```python
from build123d import *

# Parameters (mm, degrees)
SKETCH1_R           = 2.475
EXTRUDE1_DEPTH      = 17.8
SKETCH2_OUTSIDE_W   = 10.776
SKETCH2_OUTSIDE_H   = 10.776
SKETCH2_OUTSIDE_W_2 = 2.9
SKETCH2_OUTSIDE_H_2 = 7
EXTRUDE2_DEPTH      = 6
CHAMFER1_SIZE       = 0.3
CHAMFER2_SIZE       = 0.3


with BuildPart() as part:
    # Sketch1 → Extrude1 (new body)
    with BuildSketch(Plane.XY):
        Circle(SKETCH1_R)
    extrude(amount=EXTRUDE1_DEPTH)

    # Sketch2 outside → Extrude2 (cut)
    with BuildSketch(Plane.XY.offset(17.8)):
        Rectangle(SKETCH2_OUTSIDE_W, SKETCH2_OUTSIDE_H)
        Rectangle(SKETCH2_OUTSIDE_W_2, SKETCH2_OUTSIDE_H_2, mode=Mode.SUBTRACT)
    extrude(amount=-EXTRUDE2_DEPTH, mode=Mode.SUBTRACT)

    # Chamfer1
    chamfer1_edges = [part.edges().sort_by_distance(p)[0] for p in [
        (0, 2.475, 17.8),
        (0, -2.475, 17.8),
    ]]
    chamfer(chamfer1_edges, length=CHAMFER1_SIZE)

    # Chamfer2
    chamfer2_edges = [part.edges().sort_by_distance(p)[0] for p in [
        (-1.45, 0, 11.8),
        (1.45, 0, 11.8),
    ]]
    chamfer(chamfer2_edges, length=CHAMFER2_SIZE)


solid = part.part
```
Input: part model. Units: mm. Frame: model coordinates. A direction names the side the tool comes from. Round coordinates to 2 decimals unless told otherwise and drop trailing zeros. Loops run counter-clockwise (first coordinate to the right, second up) from the corner with the lowest first, then second, coordinate; pieces in that order, holes last. Notation, with made-up numbers: (48, 74.5) -> (97, 74.5) arc R15 ccw to (97, 82.5) -> close; hole circle Ø10 at (15, -5). An arc over 180 degrees is marked (long way). One line per item, written item: value.
(1) Pin query (flat end, axial travel): pin 1 (2 mm diameter, centred on y = 0, z = 16, fed in from +X); pin 2 (1 mm diameter, centred on x = 1.5, z = 2.5, fed in from +Y); pin 3 (1 mm diameter, centred on y = 1, z = 10.5, fed in from -X); pin 4 (1.5 mm diameter, centred on x = -0.5, y = 1, fed in from -Z). Return the tip coordinate at first contact, or that it passes through.
Geometry check:
pin 1: x = 1.45
pin 2: y = 2.26
pin 3: x = -2.42
pin 4: z = 0
(2) Material intervals for line 1 (X direction, y = 0.25, z = 16.5); line 2 (Z direction, x = -2.15, y = 0.3); line 3 (X direction, y = -0.1, z = 9), sorted ascending. Write a range as [from, to].
Geometry check:
line 1: [-1.45, 1.45]
line 2: [0, 11.8]
line 3: [-2.47, 2.47]
(3) Set-up query: faces 1 (the face through (-1.45, 0, 15)), 2 (the face through (2.36, 0.74, 6.68)), 3 (the face through (1.45, 0, 15)). Return all of +Z, -Z, +X, -X, +Y, -Y with unobstructed straight access to the full face (end or side cutting, diameter ignored); none if empty.
Geometry check:
face 1: +Z, -X, +Y, -Y
face 2: +Z, -Z
face 3: +Z, +X, +Y, -Y
(4) Section C-C (y = 1.45). Return the cut outline in (x, z), plus the area to 3 significant figures.
Geometry check:
outline: (-2.01, 0) -> (2.01, 0) -> (2.01, 11.8) -> (1.75, 11.8) -> (1.45, 12.1) -> (1.45, 17.8) -> (-1.45, 17.8) -> (-1.45, 12.1) -> (-1.75, 11.8) -> (-2.01, 11.8) -> close
area: 64.8 mm2
(5) Section B-B (z = 2.5). Return the cut outline in (x, y) (3 decimals).
Geometry check:
outline: circle Ø4.95 at (0, 0)
(6) Section A-A (y = 0). Return the cut outline in (x, z) (3 decimals).
Geometry check:
outline: (-2.475, 0) -> (2.475, 0) -> (2.475, 11.8) -> (1.75, 11.8) -> (1.45, 12.1) -> (1.45, 17.8) -> (-1.45, 17.8) -> (-1.45, 12.1) -> (-1.75, 11.8) -> (-2.475, 11.8) -> close
